Here's how the part is built. I have some questions about the finished solid (model axes, mm). A direction names the side the tool comes from. Give positions to 0.01 mm unless a question says otherwise; leave off trailing zeros. Order: outer loops, then holes, each group sorted by start corner. A loop starts at its lowest first (then second) coordinate and runs counter-clockwise, first axis right, second up. Notation, with made-up numbers: M 24.5,8.25 L 30.5,8.25 A18 cw 30.5,19.25 Z; hole C -9.5,24 d4. An arc over 180 degrees is marked long. Use one line per item in the form item = value.
from build123d import *

# Parameters (mm, degrees)
BOX004_W     = 36
BOX004_H     = 13
BOX004_DEPTH = 3
BOX005_W     = 25
BOX005_H     = 26
BOX005_DEPTH = 3
BOX003_W     = 71
BOX003_H     = 26
BOX003_DEPTH = 3


with BuildPart() as cube004:
    # Box004 → Box004 (new body)
    with BuildSketch(Plane(origin=(-12, 38, -107), x_dir=(1, 0, 0), z_dir=(0, 0, 1))):
        with Locations((18, 6.5)):
            Rectangle(BOX004_W, BOX004_H)
    extrude(amount=BOX004_DEPTH)


with BuildPart() as cube005:
    # Box005 → Box005 (new body)
    with BuildSketch(Plane(origin=(24, 38, -107), x_dir=(1, 0, 0), z_dir=(0, 0, 1))):
        with Locations((12.5, 13)):
            Rectangle(BOX005_W, BOX005_H)
    extrude(amount=BOX005_DEPTH)


with BuildPart() as fusion:
    # Box003 → Box003 (new body)
    with BuildSketch(Plane(origin=(-83, 38, -107), x_dir=(1, 0, 0), z_dir=(0, 0, 1))):
        with Locations((35.5, 13)):
            Rectangle(BOX003_W, BOX003_H)
    extrude(amount=BOX003_DEPTH)

    # Fusion: union Cube004, Cube005
    add(cube004.part)
    add(cube005.part)


solid = fusion.part
Q1. I want a section at B-B on z = -104.65. Write out the boundary of the cut face in (x, y).
Found:
outline = M -83,38 L 49,38 L 49,64 L 24,64 L 24,51 L -12,51 L -12,64 L -83,64 Z
Q2. I want a section at C-C on x = -3.5. Write out the boundary of the cut face in (y, z), then the cut area to 3 significant figures.
Found:
outline = M 38,-107 L 51,-107 L 51,-104 L 38,-104 Z
area = 39.0 mm²
Q3. I need wall thicknesses on L1, parallel to X at y = 59.75, z = -105; L2, parallel to Y at x = 9.5, z = -104.5. Which ranges of each line are inside material? Lowest first, please.
Found:
L1 = -83 to -12, 24 to 49
L2 = 38 to 51
Q4. On a 3-axis mill with a long thin cutter (end or side, diameter ignored), from which of +Z, -Z, +X, -X, +Y, -Y can I reach the whole of each face in a straight line? I mean faces 1 (the face through (-18, 38, -106)), 2 (the face through (24, 57, -106)). Say none if no direction works.
Found:
face_1 = +Z, -Z, +X, -X, -Y
face_2 = +Z, -Z, +Y
Q5. Thinking about a two-plate mould opening in X: for faces 3 (the face through (6, 51, -106)), 4 (the face through (-12, 57, -106)), 5 (the face through (-18, 51, -104)), 6 (the face through (49, 51, -106)), which applies, +X half, -X half, draft (parallel to the pull), parting line (faces both ways), or undercut?
Found:
face_3 = undercut
face_4 = undercut
face_5 = draft
face_6 = +X half
Q6. I want a section at A-A on y = 58. Write out the boundary of the cut face in (x, z), then the cut area to 3 significant figures.
Found:
outline = M -83,-107 L -12,-107 L -12,-104 L -83,-104 Z; M 24,-107 L 49,-107 L 49,-104 L 24,-104 Z
area = 288 mm²
